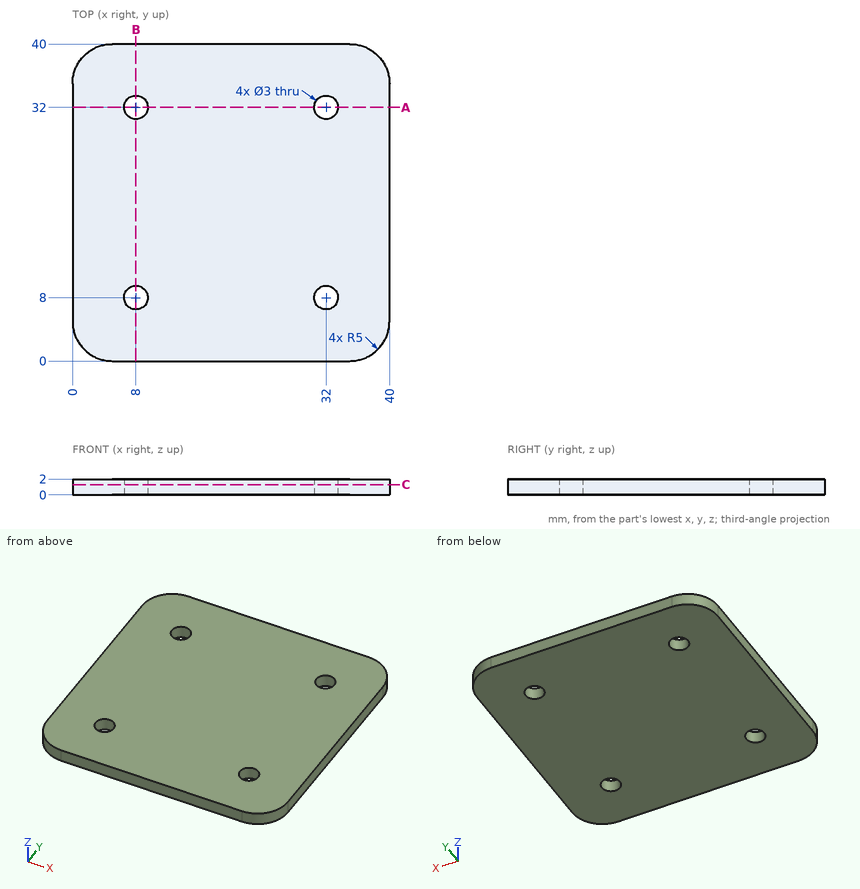
The drawing under review shows one solid part. Ordinate dimensions are in mm from its lowest x, y, z. Coordinates: 2 decimals unless noted, no trailing zeros. Write each loop counter-clockwise with the first axis right and the second up, starting at its lowest first coordinate (ties: lowest second). Pieces come first, ordered by that corner, then holes. Notation, with made-up numbers: (79, -23) - (110, -23) arc R23 ccw to (110, -6) - close; hole circle Ø3 at (-31.5, 56). An arc over 180 degrees is marked (long way). Put each result on its own line as item: value.
1. For pin 1 (1.8 mm diameter, centred on x = 32, y = 32, fed in from +Z), flat-tipped, find the tip position at first contact; note if it passes through.
Values found:
pin 1: through
2. Add section C-C, the plane z = 1.3. Give the boundary of the cut face in (x, y), then the cut area to 3 significant figures.
Values found:
outline: (0, 5) arc R5 ccw to (5, 0) - (35, 0) arc R5 ccw to (40, 5) - (40, 35) arc R5 ccw to (35, 40) - (5, 40) arc R5 ccw to (0, 35) - close; hole circle Ø3 at (8, 8); hole circle Ø3 at (8, 32); hole circle Ø3 at (32, 8); hole circle Ø3 at (32, 32)
area: 1,550 mm²
3. Wall thickness on probe 1 along X at (y, z) = (32, 0.5); probe 2 along X at (y, z) = (8.5, 0.3): over which ranges is each line inside the solid? List them lowest first.
Values found:
probe 1: 0 to 6.5, 9.5 to 30.5, 33.5 to 40
probe 2: 0 to 6.59, 9.41 to 30.59, 33.41 to 40
4. Add section A-A, the plane y = 32. Give the boundary of the cut face in (x, z).
Values found:
outline: (0, 0) - (6.5, 0) - (6.5, 2) - (0, 2) - close; (9.5, 0) - (30.5, 0) - (30.5, 2) - (9.5, 2) - close; (33.5, 0) - (40, 0) - (40, 2) - (33.5, 2) - close
